For this review, take the finished solid that the model builds, in its own axes (mm). Face numbers are marked on the shaded views. A direction names the side the tool comes from. Coordinates: 2 decimals unless noted, no trailing zeros. Loops run counter-clockwise (first coordinate to the right, second up) from the corner with the lowest first, then second, coordinate; pieces in that order, holes last. Notation, with made-up numbers: (89, -9) - (123, -9) arc R21 cw to (123, 20) - close; hole circle Ø8 at (-13, 73). An arc over 180 degrees is marked (long way). Answer as a JSON object with one key per item and string values. Group by question number.
Item 1: Tool access review of the marked faces 4, 5 and 6: name each direction out of +Z, -Z, +X, -X, +Y, -Y from which nothing blocks a thin tool from reaching the whole face with its end or side.
Item 2: To check wall thickness, follow line 1 (X direction, y = 10, z = 24); line 2 (Y direction, x = 0, z = 29); line 3 (Y direction, x = 18, z = -15). State the ranges of each line that lie inside material, in increasing order.
Item 3: We need section C-C (y = 10). Give the boundary of the cut face in (x, z).
Item 4: We need section B-B (x = -26). Give the boundary of the cut face in (y, z), then the cut area to 3 significant figures.
Item 5: We need section A-A (z = 27). Give the boundary of the cut face in (x, y), then the cut area to 3 significant figures.
Item 6: Mouldability with a two-part tool opening along Z and no side actions: class the marked faces 1, 2 and 3 as released by +Z, released by -Z, zero draft, split by the parting line, or undercut.
Item 7: We need section D-D (z = 11). Give the boundary of the cut face in (x, y), then the cut area to 3 significant figures.
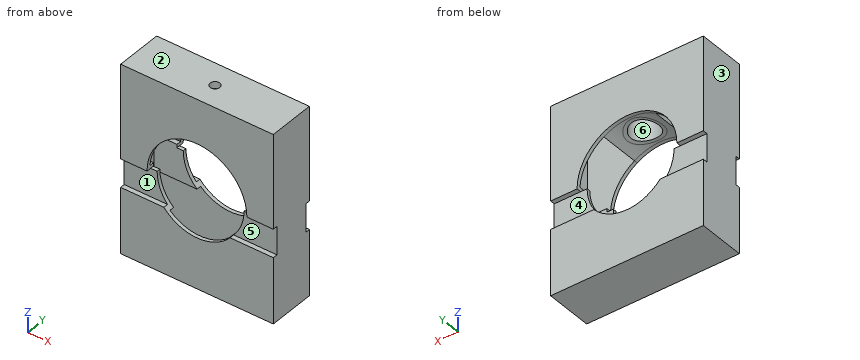
from build123d import *
from build123d.topology import SkipClean

# Parameters (mm, degrees)
SKETCH_1_W              = 65
SKETCH_1_H              = 80
EXTRUDE_1_DEPTH         = 20
CUT_EXTRUDE_1_DEPTH     = 56.283360969
SKETCH_3_R              = 18.5
CUT_EXTRUDE_2_DEPTH     = 56.283360969
SKETCH_4_R              = 6
CUT_EXTRUDE_3_DEPTH     = 37
CUT_EXTRUDE_4_REACH     = 90.635
SKETCH_5_R              = 2.1
SKETCH_6_W              = 65
SKETCH_6_H              = 12
CUT_EXTRUDE_5_DEPTH     = 2
SKETCH_7_W              = 65
SKETCH_7_H              = 12
CUT_EXTRUDE_6_DEPTH     = 2
SHELL_START             = -38.5
SHELL_1_DEPTH           = 77
SHELL_1_2_DEPTH         = 25
SHELL_START_2           = 1.5
SHELL_1_3_DEPTH         = 37
EXTRUDE_START           = 21.249883538
EXTRUDE_2_OUTLINE_W     = 22
EXTRUDE_2_OUTLINE_H     = 17
EXTRUDE_2_OUTLINE_R     = 7.5
EXTRUDE_2_OUTLINE_H_2   = 26.054315759
EXTRUDE_2_DEPTH         = 18.750116462
EXTRUDE_START_2         = 18.181377836
EXTRUDE_2_2_OUTLINE_W   = 22
EXTRUDE_2_2_OUTLINE_H   = 17
EXTRUDE_2_2_OUTLINE_H_2 = 26.054315759
EXTRUDE_2_2_DEPTH       = 3.068505702
EXTRUDE_START_3         = -26.054315759
EXTRUDE_2_3_DEPTH       = 44.554315759
SKETCH_9_W              = 21.818622164
SKETCH_9_H              = 26.054315759
CUT_EXTRUDE_7_DEPTH     = 65.583878559


with BuildPart() as part:
    # 草图1 → 凸台-拉伸1 (new body)
    with BuildSketch(Plane(origin=(0, 0, 0), x_dir=(1, 0, 0), z_dir=(0, 1, 0))):
        Rectangle(SKETCH_1_W, SKETCH_1_H)
    extrude(amount=EXTRUDE_1_DEPTH)

    # 草图2 → 切除-拉伸1 (cut, through all)
    with BuildSketch(Plane(origin=(0, 20, 0), x_dir=(1, 0, 0), z_dir=(0, 1, 0))):
        with BuildLine():
            Line((-21.25, 0), (21.25, 0))
            ThreePointArc((21.25, 0), (0, -21.25), (-21.25, 0))
        make_face()
    extrude(amount=-CUT_EXTRUDE_1_DEPTH, mode=Mode.SUBTRACT)

    # 草图3 → 切除-拉伸2 (cut, through all)
    with BuildSketch(Plane(origin=(0, 20, 0), x_dir=(-1, 0, 0), z_dir=(0, 1, 0))):
        Circle(SKETCH_3_R)
    extrude(amount=-CUT_EXTRUDE_2_DEPTH, mode=Mode.SUBTRACT)

    # 草图4 → 切除-拉伸3 (cut)
    with BuildSketch(Plane.XY):
        with Locations(Location((0, 10, 0), (0, 0, 180))):
            Circle(SKETCH_4_R)
    extrude(amount=CUT_EXTRUDE_3_DEPTH, mode=Mode.SUBTRACT)

    # 草图5 → 切除-拉伸4 (cut, up to next)
    with BuildSketch(Plane.XY.offset(40), mode=Mode.PRIVATE) as cut_extrude_4_sk1:
        with Locations((0, 10)):
            Circle(SKETCH_5_R)
    cut_extrude_4_tool1 = extrude(cut_extrude_4_sk1.sketch, amount=-CUT_EXTRUDE_4_REACH, mode=Mode.PRIVATE) & part.part
    add(cut_extrude_4_tool1.solids().sort_by_distance((0, 10, 40))[0], mode=Mode.SUBTRACT)

    # 草图6 → 切除-拉伸5 (cut)
    with BuildSketch(Plane(origin=(0, 20, 0), x_dir=(1, 0, 0), z_dir=(0, 1, 0))):
        with Locations((0, 6)):
            Rectangle(SKETCH_6_W, SKETCH_6_H)
    extrude(amount=-CUT_EXTRUDE_5_DEPTH, mode=Mode.SUBTRACT)

    # 草图7 → 切除-拉伸6 (cut)
    with BuildSketch(Plane.XZ):
        with Locations((0, -6)):
            Rectangle(SKETCH_7_W, SKETCH_7_H)
    extrude(amount=-CUT_EXTRUDE_6_DEPTH, mode=Mode.SUBTRACT)

    # 抽壳1: read off the stored shape, not the designer's step
    # 抽壳1 outline → 抽壳1 (cut)
    with BuildSketch(Plane.XY.offset(SHELL_START)):
        with BuildLine():
            Line((3.741657387, 3.5), (31, 3.5))
            Line((31, 3.5), (31, 16.5))
            Line((31, 16.5), (3.741657387, 16.5))
            ThreePointArc((3.741657387, 16.5), (7.5, 10), (3.741657387, 3.5))
        make_face()
        with BuildLine():
            Line((-31, 16.5), (-31, 3.5))
            Line((-31, 3.5), (-3.741657387, 3.5))
            ThreePointArc((-3.741657387, 3.5), (-7.5, 10), (-3.741657387, 16.5))
            Line((-3.741657387, 16.5), (-31, 16.5))
        make_face()
    extrude(amount=SHELL_1_DEPTH, mode=Mode.SUBTRACT)

    # Shell 1 2 outline → Shell 1 2 (cut)
    with BuildSketch(Plane.XY.offset(SHELL_START)):
        with BuildLine():
            Line((-31, 1.5), (31, 1.5))
            Line((31, 1.5), (31, 3.5))
            Line((31, 3.5), (3.741657387, 3.5))
            ThreePointArc((3.741657387, 3.5), (7.5, 10), (3.741657387, 16.5))
            Line((3.741657387, 16.5), (31, 16.5))
            Line((31, 16.5), (31, 18.5))
            Line((31, 18.5), (-31, 18.5))
            Line((-31, 18.5), (-31, 16.5))
            Line((-31, 16.5), (-3.741657387, 16.5))
            ThreePointArc((-3.741657387, 16.5), (-7.5, 10), (-3.741657387, 3.5))
            Line((-3.741657387, 3.5), (-31, 3.5))
            Line((-31, 3.5), (-31, 1.5))
        make_face()
    extrude(amount=SHELL_1_2_DEPTH, mode=Mode.SUBTRACT)

    # Shell 1 3 outline → Shell 1 3 (cut)
    with BuildSketch(Plane.XY.offset(SHELL_START_2)):
        with BuildLine():
            Line((-31, 1.5), (31, 1.5))
            Line((31, 1.5), (31, 3.5))
            Line((31, 3.5), (3.741657387, 3.5))
            ThreePointArc((3.741657387, 3.5), (0, 2.5), (-3.741657387, 3.5))
            Line((-3.741657387, 3.5), (-31, 3.5))
            Line((-31, 3.5), (-31, 1.5))
        make_face()
        with BuildLine():
            Line((3.741657387, 16.5), (31, 16.5))
            Line((31, 16.5), (31, 18.5))
            Line((31, 18.5), (-31, 18.5))
            Line((-31, 18.5), (-31, 16.5))
            Line((-31, 16.5), (-3.741657387, 16.5))
            ThreePointArc((-3.741657387, 16.5), (0, 17.5), (3.741657387, 16.5))
        make_face()
    extrude(amount=SHELL_1_3_DEPTH, mode=Mode.SUBTRACT)

    # 凸台-拉伸2: read off the stored shape, not the designer's step
    # 凸台-拉伸2 outline → 凸台-拉伸2 (add)
    # profile 1 of 2: a face of its own
    with BuildSketch(Plane.XY.offset(EXTRUDE_START)):
        with Locations((0, 10)):
            Rectangle(EXTRUDE_2_OUTLINE_W, EXTRUDE_2_OUTLINE_H)
        with Locations((0, 10)):
            Circle(EXTRUDE_2_OUTLINE_R, mode=Mode.SUBTRACT)
    # profile 2 of 2: a face of its own
    with BuildSketch(Plane.XY.offset(EXTRUDE_START)):
        with Locations((0, -13.02715788)):
            Rectangle(EXTRUDE_2_OUTLINE_W, EXTRUDE_2_OUTLINE_H_2)
    extrude(amount=EXTRUDE_2_DEPTH)

    # Extrude 2 2 outline → Extrude 2 2 (add)
    # profile 1 of 2: a face of its own
    with BuildSketch(Plane.XY.offset(EXTRUDE_START_2)):
        with Locations((0, 10)):
            Rectangle(EXTRUDE_2_2_OUTLINE_W, EXTRUDE_2_2_OUTLINE_H)
        with BuildLine():
            ThreePointArc((0.070228488, 2.50032881), (-5.676e-05, 2.5), (-0.070342004, 2.500329874))
            ThreePointArc((-0.070342004, 2.500329874), (-7.5, 10.000015586), (-0.070310835, 17.499670419))
            ThreePointArc((-0.070310835, 17.499670419), (-2.7611e-05, 17.5), (0.070255616, 17.499670936))
            ThreePointArc((0.070255616, 17.499670936), (7.5, 9.999986435), (0.070228488, 2.50032881))
        make_face(mode=Mode.SUBTRACT)
    # profile 2 of 2: a face of its own
    with BuildSketch(Plane.XY.offset(EXTRUDE_START_2)):
        with Locations((0, -13.02715788)):
            Rectangle(EXTRUDE_2_2_OUTLINE_W, EXTRUDE_2_2_OUTLINE_H_2)
    extrude(amount=EXTRUDE_2_2_DEPTH)

    # Extrude 2 3 outline → Extrude 2 3 (cut)
    with SkipClean():  # the faces are left unmerged after this step: merging them gives an invalid solid
        with BuildSketch(Plane(origin=(0, 0, 0), x_dir=(1, 0, 0), z_dir=(0, 1, 0)).offset(EXTRUDE_START_3)):
            with BuildLine():
                Line((11, -18.181377836), (-11, -18.181377836))
                ThreePointArc((-11, -18.181377836), (0, -21.25), (11, -18.181377836))
            make_face()
        extrude(amount=EXTRUDE_2_3_DEPTH, mode=Mode.SUBTRACT)

    # 草图9 → 切除-拉伸7 (cut, through all)
    with SkipClean():  # the faces are left unmerged after this step: merging them gives an invalid solid
        with BuildSketch(Plane(origin=(11, 0, 0), x_dir=(0, 0, -1), z_dir=(1, 0, 0))):
            with Locations((-29.090688918, -13.02715788)):
                Rectangle(SKETCH_9_W, SKETCH_9_H)
        extrude(amount=-CUT_EXTRUDE_7_DEPTH, mode=Mode.SUBTRACT)


solid = part.part
Check sheet entries:
{
 "1": {"face 4": "+X, -X, +Y", "face 5": "+X, -X, -Y", "face 6": "none"},
 "2": {"line 1": "x = -32.5 to -31, -11 to -6, 6 to 11, 31 to 32.5", "line 2": "y = 0 to 4, 16 to 20", "line 3": "y = 0 to 1.5, 18.5 to 20"},
 "3": {"outline": "(-32.5, -40) - (32.5, -40) - (32.5, 40) - (2.1, 40) - (2.1, 37) - (6, 37) - (6, 20.39) arc R21.25 cw to (11, 18.18) - (11, 38.5) - (31, 38.5) - (31, -38.5) - (-31, -38.5) - (-31, 38.5) - (-11, 38.5) - (-11, 18.18) arc R21.25 cw to (-6, 20.39) - (-6, 37) - (-2.1, 37) - (-2.1, 40) - (-32.5, 40) - close"},
 "4": {"outline": "(0, -40) - (20, -40) - (20, -12) - (18, -12) - (18, 0) - (20, 0) - (20, 40) - (0, 40) - (0, 0) - (2, 0) - (2, -12) - (0, -12) - close; hole (1.5, -38.5) - (18.5, -38.5) - (18.5, -13.5) - (16.5, -13.5) - (16.5, 1.5) - (18.5, 1.5) - (18.5, 38.5) - (1.5, 38.5) - (1.5, 1.5) - (3.5, 1.5) - (3.5, -13.5) - (1.5, -13.5) - close", "area": "303 mm2"},
 "5": {"outline": "(-32.5, 0) - (32.5, 0) - (32.5, 20) - (-32.5, 20) - close; hole (-31, 1.5) - (-11, 1.5) - (-11, 18.5) - (-31, 18.5) - close; hole circle Ø12 at (0, 10); hole (11, 1.5) - (31, 1.5) - (31, 18.5) - (11, 18.5) - close", "area": "507 mm2"},
 "6": {"face 1": "undercut", "face 2": "released by +Z", "face 3": "zero draft"},
 "7": {"outline": "(-32.5, 0) - (-18.18, 0) - (-18.18, 1.5) - (-31, 1.5) - (-31, 18.5) - (-18.18, 18.5) - (-18.18, 20) - (-32.5, 20) - close; (18.18, 0) - (32.5, 0) - (32.5, 20) - (18.18, 20) - (18.18, 18.5) - (31, 18.5) - (31, 1.5) - (18.18, 1.5) - close", "area": "137 mm2"}
}
